Geometry: final body of the model. Coordinates: model frame, mm. Face numbers are marked on the shaded views. Give positions to 0.01 mm unless a question says otherwise; leave off trailing zeros. Write each loop counter-clockwise with the first axis right and the second up, starting at its lowest first coordinate (ties: lowest second). Pieces come first, ordered by that corner, then holes. Notation, with made-up numbers: (-24, -8.5) -> (20, -8.5) arc R12 cw to (20, 2.5) -> close; hole circle Ø2 at (70, 7.5). An arc over 180 degrees is marked (long way). Answer as a JSON object with one key per item and string values. Group by question number.
(1) Section query B-B on z = -2. Output: boundary loops of the cut face in (x, y), plus the area to 3 significant figures.
(2) Material intervals for probe 1 along X at (y, z) = (17, 1.2); probe 2 along Y at (x, z) = (0.5, -7); probe 3 along Y at (x, z) = (35.9, 0.95), sorted ascending.
(3) Section query C-C on x = 15. Output: boundary loops of the cut face in (y, z), plus the area to 3 significant figures.
(4) Contact query for flat-ended pins moving along their axis: pin 1 Ø2 at (y, z) = (-13, -6) entering from +X; pin 2 Ø2 at (y, z) = (-15.5, -7.5) entering from -X; pin 3 Ø2.5 at (x, y) = (-35.9, 17) entering from -Z; pin 4 Ø3 at (x, z) = (-12.5, -6.5) entering from -Y. Output: stop coordinate, or through.
(5) Section query D-D on y = 25. Output: boundary loops of the cut face in (x, z), plus the area to 3 significant figures.
(6) Section query A-A on x = 35.9. Output: boundary loops of the cut face in (y, z).
(7) Draft query along Y for the marked faces 1, 2 and 3. Return one class per face: +Y half, -Y half, draft (parallel to the pull), parting line (faces both ways), or undercut.
from build123d import *

# Parameters (mm, degrees)
SKETCH1_W           = 79.8
SKETCH1_H           = 70
BOSS_EXTRUDE1_DEPTH = 1.7
SKETCH1_3_W         = 55
SKETCH1_3_H         = 2.5
BOSS_EXTRUDE2_DEPTH = 9.5
SKETCH1_4_R         = 1.65
CUT_EXTRUDE1_DEPTH  = 54.919013344


with BuildPart() as part:
    # Sketch1 → Boss-Extrude1 (new body)
    with BuildSketch(Plane.XY):
        Rectangle(SKETCH1_W, SKETCH1_H)
    extrude(amount=BOSS_EXTRUDE1_DEPTH)

    # Sketch1_3 → Boss-Extrude2 (add)
    with BuildSketch(Plane.XY):
        with Locations((0, -12.7)):
            Rectangle(SKETCH1_3_W, SKETCH1_3_H)
        with Locations((0, 12.7)):
            Rectangle(SKETCH1_3_W, SKETCH1_3_H)
        with Locations((0, -17.7)):
            Rectangle(SKETCH1_3_W, SKETCH1_3_H)
        with Locations((0, 17.7)):
            Rectangle(SKETCH1_3_W, SKETCH1_3_H)
    extrude(amount=-BOSS_EXTRUDE2_DEPTH)

    # Sketch1_4 → Cut-Extrude1 (cut, through all)
    with BuildSketch(Plane.XY):
        with Locations((-35.9, 17)):
            Circle(SKETCH1_4_R)
        with Locations(Location((35.9, 17, 0), (0, 0, 180))):
            Circle(SKETCH1_4_R)
        with Locations((35.9, -17)):
            Circle(SKETCH1_4_R)
        with Locations(Location((-35.9, -17, 0), (0, 0, 180))):
            Circle(SKETCH1_4_R)
    extrude(amount=CUT_EXTRUDE1_DEPTH, mode=Mode.SUBTRACT)


solid = part.part
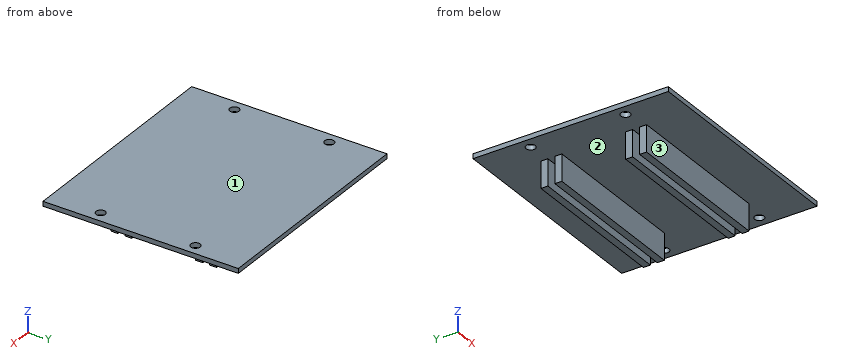
Answer list:
{
 "1": {"outline": "(-27.5, -18.95) -> (27.5, -18.95) -> (27.5, -16.45) -> (-27.5, -16.45) -> close; (-27.5, -13.95) -> (27.5, -13.95) -> (27.5, -11.45) -> (-27.5, -11.45) -> close; (-27.5, 11.45) -> (27.5, 11.45) -> (27.5, 13.95) -> (-27.5, 13.95) -> close; (-27.5, 16.45) -> (27.5, 16.45) -> (27.5, 18.95) -> (-27.5, 18.95) -> close", "area": "550 mm2"},
 "2": {"probe 1": "-39.9 to -37.55, -34.25 to 34.25, 37.55 to 39.9", "probe 2": "-18.95 to -16.45, -13.95 to -11.45, 11.45 to 13.95, 16.45 to 18.95", "probe 3": "-35 to -18.65, -15.35 to 15.35, 18.65 to 35"},
 "3": {"outline": "(-35, 0) -> (-18.95, 0) -> (-18.95, -9.5) -> (-16.45, -9.5) -> (-16.45, 0) -> (-13.95, 0) -> (-13.95, -9.5) -> (-11.45, -9.5) -> (-11.45, 0) -> (11.45, 0) -> (11.45, -9.5) -> (13.95, -9.5) -> (13.95, 0) -> (16.45, 0) -> (16.45, -9.5) -> (18.95, -9.5) -> (18.95, 0) -> (35, 0) -> (35, 1.7) -> (-35, 1.7) -> close", "area": "214 mm2"},
 "4": {"pin 1": "x = 27.5", "pin 2": "x = -27.5", "pin 3": "through", "pin 4": "y = -18.95"},
 "5": {"outline": "(-39.9, 0) -> (39.9, 0) -> (39.9, 1.7) -> (-39.9, 1.7) -> close", "area": "136 mm2"},
 "6": {"outline": "(-35, 0) -> (-18.65, 0) -> (-18.65, 1.7) -> (-35, 1.7) -> close; (-15.35, 0) -> (15.35, 0) -> (15.35, 1.7) -> (-15.35, 1.7) -> close; (18.65, 0) -> (35, 0) -> (35, 1.7) -> (18.65, 1.7) -> close"},
 "7": {"face 1": "draft", "face 2": "undercut", "face 3": "-Y half"}
}
